```python
from build123d import *

# Parameters (mm, degrees)
F0_W       = 85.0676417184
F0_H       = 115.57
F1_DEPTH   = 6.35
F2_R       = 12.4631910905
F3_DEPTH   = 6.351
F1_FACE1_W = 85.0676417184
F1_FACE1_H = 115.57
F1_FACE1_R = 12.4631910905
F4_W       = 85.0676417184
F4_H       = 115.57
F4_R       = 12.4631910905
F4_R_2     = 12.0047888383
F5_DEPTH   = 25.4


with BuildPart() as f1:
    # F0 (on Top) → F1 (new body)
    with BuildSketch(Plane.XY):
        Rectangle(F0_W, F0_H)
    extrude(amount=F1_DEPTH)

    # F2 (on Top) → F3 (cut, through all)
    with BuildSketch(Plane.XY):
        Circle(F2_R)
    extrude(amount=F3_DEPTH, mode=Mode.SUBTRACT)

    # F1_face1 (on face) + F4 (on face) → F5 (join)
    with BuildSketch(Plane(origin=(0, 0, 0), x_dir=(1, 0, 0), z_dir=(0, 0, -1))):
        Rectangle(F1_FACE1_W, F1_FACE1_H)
        Circle(F1_FACE1_R, mode=Mode.SUBTRACT)
    with BuildSketch(Plane.XY.offset(6.35)):
        Rectangle(F4_W, F4_H)
        Circle(F4_R, mode=Mode.SUBTRACT)
        with Locations((30.233990401, 0)):
            Circle(F4_R_2, mode=Mode.SUBTRACT)
    extrude(amount=F5_DEPTH, dir=(0, 0, -1))


solid = f1.part
```
CAD build for the part. Positions are in the model's coordinates, mm. Give positions to 0.01 mm unless a question says otherwise; leave off trailing zeros. Write each loop counter-clockwise with the first axis right and the second up, starting at its lowest first coordinate (ties: lowest second). Pieces come first, ordered by that corner, then holes. Notation, with made-up numbers: M 40.25,1.5 L 51.25,1.5 A33 ccw 51.25,33.5 Z; hole C 10.5,87.5 d3. An arc over 180 degrees is marked long. Return JSON: item names as keys, results as strings. Group by question number.
(1) Band-saw the part on B-B (y = 0). Give the cut face in (x, z), and give its area (3 significant figures).
(2) Drill centre lines: L1, parallel to X at y = 0, z = -12.5; L2, parallel to Y at x = 0, z = -7 (3 decimals); L3, parallel to X at y = -9, z = 1. Where is each one in solid material? Low to high. Write a range as [from, to].
(3) Band-saw the part on A-A (x = 0). Give the cut face in (y, z) (3 decimals), and give its area (3 significant figures).
(4) Flat gauge pin, fed straight in: pin 1 Ø15 at (x, y) = (0, 0) entering from +Z. Where does the tip first touch, or does it go through?
(5) Band-saw the part on C-C (z = -2.5). Give the cut face in (x, y) (3 decimals), and give its area (3 significant figures).
(6) Mould opens along X. For faces 1 (the face through (-1, 14, 6.35)), 2 (the face through (-42.534, 1, -9)), 3 (the face through (-2.702, -12.167, -9.747)), 4 (the face through (42.534, 1, -9)) say: pulls with the +X half, pulls with the -X half, needs draft (parallel to the pull), parting line crosses it, or undercut.
Entries:
{
 "1": {"outline": "M -42.53,-25.4 L -12.46,-25.4 L -12.46,6.35 L -42.53,6.35 Z; M 12.46,-25.4 L 42.53,-25.4 L 42.53,6.35 L 12.46,6.35 Z", "area": "1,910 mm^2"},
 "2": {"L1": "x = [-42.53, -12.46], [12.46, 42.53]", "L2": "y = [-57.785, -12.463], [12.463, 57.785]", "L3": "x = [-42.53, -8.62], [8.62, 42.53]"},
 "3": {"outline": "M -57.785,-25.4 L -12.463,-25.4 L -12.463,6.35 L -57.785,6.35 Z; M 12.463,-25.4 L 57.785,-25.4 L 57.785,6.35 L 12.463,6.35 Z", "area": "2,880 mm^2"},
 "4": {"pin 1": "passes through"},
 "5": {"outline": "M -42.534,-57.785 L 42.534,-57.785 L 42.534,57.785 L -42.534,57.785 Z; hole C 0,0 d24.926", "area": "9,340 mm^2"},
 "6": {"face 1": "needs draft", "face 2": "pulls with the -X half", "face 3": "undercut", "face 4": "pulls with the +X half"}
}
